Work out the finished part from the listing and answer in its coordinate system (mm). Face numbers are marked on the shaded views. A direction names the side the tool comes from. Coordinates: 2 decimals unless noted, no trailing zeros. Write each loop counter-clockwise with the first axis right and the second up, starting at its lowest first coordinate (ties: lowest second). Pieces come first, ordered by that corner, then holes. Notation, with made-up numbers: (21.25, 85) - (80.25, 85) arc R26 ccw to (80.25, 100) - close; hole circle Ø1 at (-35, 53.5). An arc over 180 degrees is marked (long way). Use a Markdown table: item, result. Add a question column.
(1) The part is cut by section C-C, the plane x = -20. Give the vertices of the cut face in (y, z).
(2) For a pull along X with two mould halves and no side action, classify the marked faces 1, 2 and 3 as released by +X, released by -X, zero draft, split by the parting line, or undercut.
(3) The part is cut by section B-B, the plane y = 7.5. Give the vertices of the cut face in (x, z) (3 decimals), then the cut area to 3 significant figures.
(4) A tool of negligible diameter and unlimited length cuts with its end or side. For the marked faces 4, 5, 6 and 7, from which of +Z, -Z, +X, -X, +Y, -Y can it reach the whole face along a straight path? Write none if from no direction.
(5) Given pin 1 Ø4 at (y, z) = (6, 3) entering from -X; pin 2 Ø1.5 at (x, y) = (-9, 5.5) entering from +Z; pin 3 Ø3 at (y, z) = (12.5, 3) entering from +X, each flat-ended and moving along its own axis, determine where each tip first touches the part or whether it passes through.
(6) The part is cut by section A-A, the plane z = 0. Give the vertices of the cut face in (x, y) (3 decimals).
(7) The part is cut by section D-D, the plane z = 25. Give the vertices of the cut face in (x, y).
(8) Find the intervals of material crossed by line 1 (X direction, y = 3, z = 0) (3 decimals); line 2 (X direction, y = 11.3, z = 0); line 3 (Z direction, x = 0, y = 3.25) (3 decimals), in increasing order. Write a range as from..to.
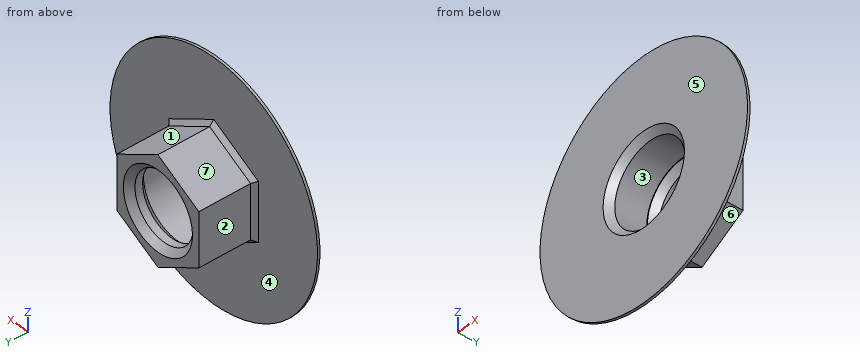
from build123d import *

# Parameters (mm, degrees)
SKETCH1_R                       = 27
SKETCH1_R_2                     = 9.675
BOSS_EXTRUDE1_DEPTH             = 0.6
SKETCH2_R                       = 9.675
BOSS_EXTRUDE2_DEPTH             = 13.5
SKETCH3_R                       = 10.043523413
SKETCH3_R_2                     = 8
BOSS_EXTRUDE3_DEPTH             = 4.85
CHAMFER1_SIZE                   = 1.5
SKETCH4_R                       = 28.5
SKETCH4_R_2                     = 25
BOSS_EXTRUDE4_DEPTH             = 1.9
BOSS_EXTRUDE4_DIRECTION_2_REACH = 42.704
CHAMFER3_SIZE                   = 1
CUT_EXTRUDE1_START              = -1.9
SKETCH5_R                       = 28.5
CUT_EXTRUDE1_DEPTH              = 1.9


with BuildPart() as part:
    # Sketch1 → Boss-Extrude1 (new body)
    with BuildSketch(Plane(origin=(0, 0, 0), x_dir=(1, 0, 0), z_dir=(0, 1, 0))):
        with Locations(Location((0, 0, 0), (0, 0, 270))):
            Circle(SKETCH1_R)
        with Locations(Location((0, 0, 0), (0, 0, 270))):
            Circle(SKETCH1_R_2, mode=Mode.SUBTRACT)
    extrude(amount=BOSS_EXTRUDE1_DEPTH)

    # Sketch2 → Boss-Extrude2 (add)
    with BuildSketch(Plane(origin=(0, 0.6, 0), x_dir=(1, 0, 0), z_dir=(0, 1, 0))):
        Polygon((0, 12.990381057), (-11.25, 6.495190528), (-11.25, -6.495190528), (0, -12.990381057), (11.25, -6.495190528), (11.25, 6.495190528), align=None)
        with Locations(Location((0, 0, 0), (0, 0, 270))):
            Circle(SKETCH2_R, mode=Mode.SUBTRACT)
    extrude(amount=BOSS_EXTRUDE2_DEPTH)

    # Sketch3 → Boss-Extrude3 (add)
    with BuildSketch(Plane(origin=(0, 14.1, 0), x_dir=(1, 0, 0), z_dir=(0, 1, 0))):
        Circle(SKETCH3_R)
        with Locations(Location((0, 0, 0), (0, 0, 270))):
            Circle(SKETCH3_R_2, mode=Mode.SUBTRACT)
    extrude(amount=-BOSS_EXTRUDE3_DEPTH)

    # Chamfer1
    chamfer1_edges = [part.edges().sort_by_distance(p)[0] for p in [
        (0, 9.25, -8),
        (0, 14.1, -8),
        (0, 0, -9.675),
    ]]
    chamfer(chamfer1_edges, length=CHAMFER1_SIZE)

    # Sketch4 → Boss-Extrude4 (add)
    with BuildSketch(Plane.XZ):
        with Locations(Location((0, 0, 0), (0, 0, 270))):
            Circle(SKETCH4_R)
        with Locations(Location((0, 0, 0), (0, 0, 270))):
            Circle(SKETCH4_R_2, mode=Mode.SUBTRACT)
    extrude(amount=BOSS_EXTRUDE4_DEPTH)

    # Boss-Extrude4 direction 2: up to this face of the body (flat: up to its plane)
    boss_extrude4_direction_2_end = Plane(part.part.faces().sort_by_distance((0, 0.6, -26.236324676))[0])
    # Sketch4 → Boss-Extrude4 direction 2 (add, up to the picked face)
    with BuildSketch(Plane.XZ, mode=Mode.PRIVATE) as boss_extrude4_direction_2_sk1:
        with Locations(Location((0, 0, 0), (0, 0, 270))):
            Circle(SKETCH4_R)
        with Locations(Location((0, 0, 0), (0, 0, 270))):
            Circle(SKETCH4_R_2, mode=Mode.SUBTRACT)
    boss_extrude4_direction_2_tool1 = split(extrude(boss_extrude4_direction_2_sk1.sketch, amount=-BOSS_EXTRUDE4_DIRECTION_2_REACH, mode=Mode.PRIVATE), bisect_by=boss_extrude4_direction_2_end, keep=Keep.BOTH, mode=Mode.PRIVATE)
    add(boss_extrude4_direction_2_tool1.solids().sort_by(Axis((0, 0, 27.693898), (0, 1, 0)))[0])

    # Chamfer3
    chamfer3_edges = [part.edges().sort_by_distance(p)[0] for p in [
        (5.625, 0.6, -9.742785793),
        (-5.625, 0.6, -9.742785793),
        (-11.25, 0.6, 0),
        (-5.625, 0.6, 9.742785793),
        (5.625, 0.6, 9.742785793),
        (11.25, 0.6, 0),
    ]]
    chamfer(chamfer3_edges, length=CHAMFER3_SIZE)

    # Sketch5 → Cut-Extrude1 (cut)
    with BuildSketch(Plane.XZ.offset(1.9).offset(CUT_EXTRUDE1_START)):
        with Locations(Location((0, 0, 0), (0, 0, 90))):
            Circle(SKETCH5_R)
    extrude(amount=CUT_EXTRUDE1_DEPTH, mode=Mode.SUBTRACT)


solid = part.part
Model answer:
| question | item | result |
|---|---|---|
| 1 | outline | (0, -20.3) - (0.6, -20.3) - (0.6, 20.3) - (0, 20.3) - close |
| 2 | face 1 | released by +X |
| 2 | face 2 | released by -X |
| 2 | face 3 | undercut |
| 3 | outline | (-11.25, -6.495) - (0, -12.99) - (11.25, -6.495) - (11.25, 6.495) - (0, 12.99) - (-11.25, 6.495) - close; hole circle Ø19.35 at (0, 0) |
| 3 | area | 144 mm^2 |
| 4 | face 4 | +Y |
| 4 | face 5 | +Z, -Z, +X, -X, -Y |
| 4 | face 6 | -Z, +X, +Y |
| 4 | face 7 | +Z, -X, +Y |
| 5 | pin 1 | x = -11.25 |
| 5 | pin 2 | z = 8.23 |
| 5 | pin 3 | x = 11.25 |
| 6 | outline | (-28.5, 0) - (-11.175, 0) - (-9.675, 1.5) - (-9.675, 9.25) - (-9.5, 9.25) - (-8, 10.75) - (-8, 12.6) - (-9.5, 14.1) - (-11.25, 14.1) - (-11.25, 1.6) - (-12.25, 0.6) - (-28.5, 0.6) - close; (8, 10.75) - (9.5, 9.25) - (9.675, 9.25) - (9.675, 1.5) - (11.175, 0) - (28.5, 0) - (28.5, 0.6) - (12.25, 0.6) - (11.25, 1.6) - (11.25, 14.1) - (9.5, 14.1) - (8, 12.6) - close |
| 7 | outline | (-13.68, 0) - (13.68, 0) - (13.68, 0.6) - (-13.68, 0.6) - close |
| 8 | line 1 | -11.25..-9.675, 9.675..11.25 |
| 8 | line 2 | -11.25..-8, 8..11.25 |
| 8 | line 3 | -12.99..-9.675, 9.675..12.99 |
